Autodesk Inventor part; units mm, degrees
ref_plane "YZ Plane" through (0, 0, 0) normal (1, 0, 0) x (0, 1, 0)
ref_plane "XZ Plane" through (0, 0, 0) normal (0, 1, 0) x (-1, 0, 0)
ref_plane "XY Plane" through (0, 0, 0) normal (0, 0, 1) x (1, 0, 0)
sketch "スケッチ1" plane through (0, 0, 0) normal (0, 0, 1) x (1, 0, 0)
  line L0 (0, 0) -> (239.9998, 0)
  line L1 (239.9998, 0) -> (239.9998, 239.9998)
  line L2 (239.9998, 239.9998) -> (0, 239.9998)
  line L3 (0, 239.9998) -> (0, 0)
  line L4 (0, 239.9998) -> (239.9998, 0)
  line L5 (-178.706, 178.706) -> (151.9787, -151.9787)
  dimension "d16" = 45
  dimension "d17" = 169.7055
extrude "プレート1" add sketch "スケッチ1" along normal blind 3 contours L3 L4 L0
sketch "スケッチ2" plane through (0, 0, 3) normal (0, 0, 1) x (1, 0, 0)
  line L0 (90, 33.5) -> (110, 33.5)
  line L1 (110, 33.5) -> (110, 86.5)
  line L2 (110, 86.5) -> (90, 86.5)
  line L3 (90, 86.5) -> (90, 33.5)
  line L4 (90, 33.5) -> (110, 86.5) construction
  line L5 (110, 33.5) -> (90, 86.5) construction
  line L6 (239.9998, 0) -> (0, 0)
  line L7 (0, 0) -> (0, 239.9998)
  line L8 (134, 30) -> (66, 30)
  line L9 (66, 30) -> (66, 90)
  line L10 (66, 90) -> (134, 90)
  line L11 (134, 90) -> (134, 30)
  line L12 (134, 30) -> (66, 90) construction
  line L13 (66, 30) -> (134, 90) construction
  point P0 (100, 60)
  dimension "d3" = 20
  dimension "d4" = 53
  dimension "d5" = 60
  dimension "d6" = 100
  dimension "d14" = 60
  dimension "d15" = 68
hole "穴1" at (90, 33.5, 3) at (110, 33.5, 3) at (90, 86.5, 3) at (110, 86.5, 3) at (66, 30, 3) at (134, 30, 3) at (66, 90, 3) direction (0, 0, -1) diameter 5.2 depth 3 tip angle 118
fillet "フィレット1" radius 2 3 edges at (0, 239.9998, 1.5) (0, 0, 1.5) (239.9998, 0, 1.5)
sketch "スケッチ3" plane through (0, 0, 3) normal (0, 0, 1) x (1, 0, 0)
  circle A0 centre (66, 90) radius 2.6
  line L0 (0, 2) -> (0, 235.1714)
  point P0 (0, 0)
  point P1 (90, 117)
  point P2 (80, 117)
  dimension "d19" = 10
  dimension "d20" = 27
  dimension "d21" = 80
hole "穴2" at (90, 117, 3) at (80, 117, 3) direction (0, 0, -1) diameter 3.242 depth 11.8 tip angle 118
sketch "スケッチ4" plane through (0, 0, 3) normal (0, 0, 1) x (1, 0, 0)
  circle A0 centre (90, 117) radius 1.621
  circle A1 centre (80, 117) radius 1.621
  arc A2 (235.1714, 0) -> (236.5856, 3.4142) centre (235.1714, 2) ccw
  line L0 (3.4142, 236.5856) -> (236.5856, 3.4142)
  arc A3 (3.4142, 236.5856) -> (0, 235.1714) centre (2, 235.1714) ccw
  line L1 (0, 2) -> (0, 235.1714)
  arc A4 (0, 2) -> (2, 0) centre (2, 2) ccw
  line L2 (235.1714, 0) -> (2, 0)
  circle A5 centre (134, 30) radius 2.6
  circle A6 centre (110, 86.5) radius 2.6
  circle A7 centre (110, 33.5) radius 2.6
  circle A8 centre (90, 33.5) radius 2.6
  circle A9 centre (90, 86.5) radius 2.6
  circle A10 centre (66, 30) radius 2.6
  circle A11 centre (66, 90) radius 2.6
  line L3 (10, 10) -> (10, 215.8577)
  line L4 (10, 215.8577) -> (215.8577, 10)
  line L5 (215.8577, 10) -> (10, 10)
  point P0 (0, 0)
  point P1 (205, 10)
  point P2 (35, 10)
  point P3 (10, 35)
  point P4 (10, 205)
  point P5 (120, 10)
  point P6 (10, 120)
  dimension "d29" = 10
  dimension "d30" = 25
  dimension "d31" = 25
  dimension "d32" = 170
  dimension "d33" = 170
  dimension "d34" = 85
  dimension "d35" = 85
hole "穴3" at (205, 10, 3) at (35, 10, 3) at (10, 35, 3) at (10, 205, 3) at (120, 10, 3) at (10, 120, 3) direction (0, 0, -1) diameter 4.2 depth 3 tip angle 118
sketch "スケッチ6" plane through (0, 0, 3) normal (0, 0, 1) x (1, 0, 0)
  circle A0 centre (120, 10) radius 2.1
  circle A1 centre (10, 35) radius 2.1
  circle A2 centre (205, 10) radius 2.1
  circle A3 centre (35, 10) radius 2.1
  circle A4 centre (10, 205) radius 2.1
  circle A5 centre (10, 120) radius 2.1
  circle A6 centre (90, 117) radius 1.621
  circle A7 centre (80, 117) radius 1.621
  arc A8 (235.1714, 0) -> (236.5856, 3.4142) centre (235.1714, 2) ccw
  line L0 (3.4142, 236.5856) -> (236.5856, 3.4142)
  arc A9 (3.4142, 236.5856) -> (0, 235.1714) centre (2, 235.1714) ccw
  line L1 (0, 2) -> (0, 235.1714)
  arc A10 (0, 2) -> (2, 0) centre (2, 2) ccw
  line L2 (235.1714, 0) -> (2, 0)
  circle A11 centre (134, 30) radius 2.6
  circle A12 centre (110, 86.5) radius 2.6
  circle A13 centre (110, 33.5) radius 2.6
  circle A14 centre (90, 33.5) radius 2.6
  circle A15 centre (90, 86.5) radius 2.6
  circle A16 centre (66, 30) radius 2.6
  circle A17 centre (66, 90) radius 2.6
  line L3 (20, 20) -> (20, 191.7155)
  line L4 (20, 191.7155) -> (191.7155, 20)
  line L5 (191.7155, 20) -> (20, 20)
  point P0 (0, 0)
  point P1 (30, 30)
  dimension "d46" = 20
  dimension "d47" = 10
  dimension "d48" = 10
hole "穴4" at (30, 30, 3) direction (0, 0, -1) diameter 5.2 depth 3 tip angle 118
equation "\"d12\" = Thickness"
equation "\"d41\" = Thickness"
equation "\"d54\" = Thickness"
equation "\"d2\" = Thickness"
equation "\"BendRadius\" = Thickness"
equation "\"BendReliefWidth\" = Thickness"
equation "\"BendReliefDepth\" = 0.5 * Thickness"
equation "\"CornerReliefSize\" = 4 * Thickness"
equation "\"MinimumRemnant\" = 2 * Thickness"
equation "\"TransitionRadius\" = BendRadius"
equation "\"JacobiRadiusSize\" = BendRadius"
equation "\"GapSize\" = Thickness"
properties part number "Display_CCM_Mount"
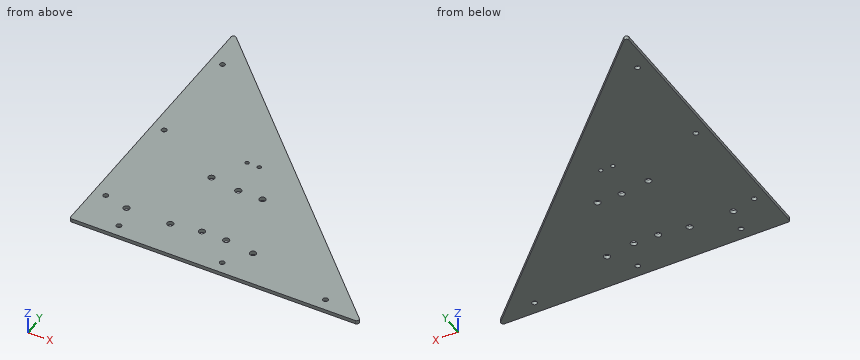
Could you check a few things on this model? Use its own coordinates, in mm. Round coordinates to 2 decimals unless told otherwise and drop trailing zeros. Loops run counter-clockwise (first coordinate to the right, second up) from the corner with the lowest first, then second, coordinate; pieces in that order, holes last. Notation, with made-up numbers: (-20, 22.25) - (25, 22.25) arc R16 cw to (25, 30.25) - close; hole circle Ø8 at (19.5, 67.5). An arc over 180 degrees is marked (long way). Write item = value, one per line.
1) Imagine slicing it at A-A (z = 0.6). Give the number of separate pieces and of enclosed holes in the cut face, and give its area (3 significant figures).
Computed:
separate_pieces = 1
enclosed_holes = 16
area = 28,500 mm2
2) Imagine slicing it at B-B (x = 57.5). Please give me the cut outline in (y, z), and give its area (4 significant figures).
Computed:
outline = (0, 0) - (182.5, 0) - (182.5, 3) - (0, 3) - close
area = 547.5 mm2
3) Imagine slicing it at C-C (y = 172.5). Please give me the cut outline in (x, z), and give its area (4 significant figures).
Computed:
outline = (0, 0) - (67.5, 0) - (67.5, 3) - (0, 3) - close
area = 202.5 mm2
4) I need wall thicknesses on line 1 along Y through (x, z) = (10, 1.45); line 2 along Y through (x, z) = (90, 1.9); line 3 along X through (y, z) = (117, 0.65). Which ranges of each line are inside material? Lowest first, please. Write a range as from..to.
Computed:
line_1 = 0..32.9, 37.1..117.9, 122.1..202.9, 207.1..230
line_2 = 0..30.9, 36.1..83.9, 89.1..115.38, 118.62..150
line_3 = 0..78.38, 81.62..88.38, 91.62..123
5) I'm going to push a flat-ended pin straight in: P1, Ø3, axis at x = 90, y = 63.5, coming from the -Z side. Where does the tip first touch, or does it pass through?
Computed:
P1 = 0
